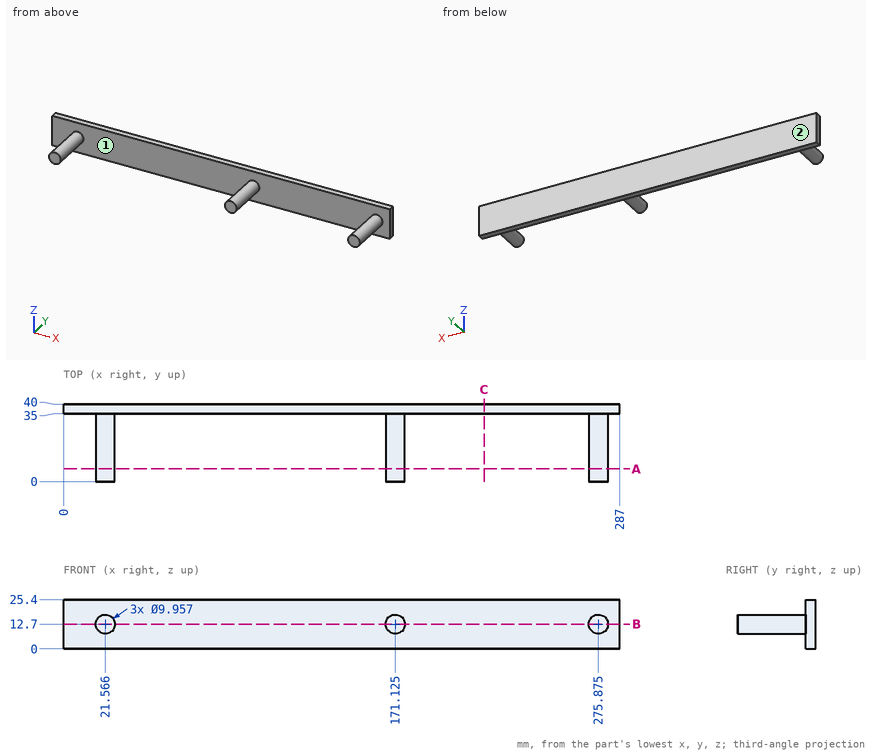
Study the drawing (mm; zero at the part's minimum x, y, z) and answer. Coordinates: 2 decimals unless noted, no trailing zeros. Write each loop counter-clockwise with the first axis right and the second up, starting at its lowest first coordinate (ties: lowest second). Pieces come first, ordered by that corner, then holes. Notation, with made-up numbers: (54, -10) - (87, -10) arc R19 cw to (87, 24) - close; hole circle Ø6 at (19.5, -7.75). An arc over 180 degrees is marked (long way). One line per item, written item: value.
1) Consider line 1 along X through (y, z) = (25.5, 13.5); line 2 along X through (y, z) = (22, 15.5); line 3 along Y through (x, z) = (78.5, 19). Determine where each line is inside the solid, lowest interval first. Write a range as from..to.
Geometry check:
line 1: x = 16.65..26.48, 166.21..176.04, 270.96..280.79
line 2: x = 17.45..25.68, 167.01..175.24, 271.76..279.99
line 3: y = 35..40
2) Find section B-B (z = 12.7). Give the vertices of the cut face in (x, y), and give its area (3 significant figures).
Geometry check:
outline: (0, 35) - (16.59, 35) - (16.59, 0) - (26.54, 0) - (26.54, 35) - (166.15, 35) - (166.15, 0) - (176.1, 0) - (176.1, 35) - (270.9, 35) - (270.9, 0) - (280.85, 0) - (280.85, 35) - (287, 35) - (287, 40) - (0, 40) - close
area: 2,480 mm2
3) Each of these flat-tipped pins is pushed along its axis until it touches: pin 1 Ø8 at (x, z) = (82.5, 22.5) entering from -Y; pin 2 Ø1 at (y, z) = (22.5, 11) entering from -X; pin 3 Ø10 at (y, z) = (9.5, 8.5) entering from -X. Where does it stop, or does it pass through?
Geometry check:
pin 1: stops at y = 35
pin 2: stops at x = 16.73
pin 3: stops at x = 16.59
4) For a pull along X with two mould halves and no side action, classify the marked faces 1 and 2 as pulls with the +X half, pulls with the -X half, needs draft (parallel to the pull), parting line crosses it, or undercut.
Geometry check:
face 1: undercut
face 2: needs draft
5) Find section C-C (x = 217). Give the vertices of the cut face in (y, z), and give its area (3 significant figures).
Geometry check:
outline: (35, 0) - (40, 0) - (40, 25.4) - (35, 25.4) - close
area: 127 mm2
6) Find section A-A (y = 6.5). Give the vertices of the cut face in (x, z) (1 decimal).
Geometry check:
outline: circle Ø10 at (21.6, 12.7); circle Ø10 at (171.1, 12.7); circle Ø10 at (275.9, 12.7)
